Verification items for the finished model (mm, model axes). A direction names the side the tool comes from. Give positions to 0.01 mm unless a question says otherwise; leave off trailing zeros. Loops run counter-clockwise (first coordinate to the right, second up) from the corner with the lowest first, then second, coordinate; pieces in that order, holes last. Notation, with made-up numbers: M 89,70 L 104,70 A24 cw 104,107 Z; hole C 48.5,80 d5. An arc over 180 degrees is marked long. Use a Markdown table: item, result.
from build123d import *

# Parameters (mm, degrees)
F_2_6_MM_REMOVABLE_SHELF_WIRING_NOTC_2_R       = 1.65
F_2_6_MM_REMOVABLE_SHELF_WIRING_NOTC_2_R_2     = 1.15
F_2_6_MM_REMOVABLE_SHELF_WIRING_NOTCH_AN_DEPTH = 2.6
CONTROLLER_START                               = 2.6
CONTROLLER_BOARD_EDGE_RESTS_PROFILE_W          = 60
CONTROLLER_BOARD_EDGE_RESTS_PROFILE_H          = 1.6
CONTROLLER_BOARD_EDGE_RESTS_DEPTH              = 2


with BuildPart() as part:
    # 2.6 mm removable shelf - wiring notc 2 → 2.6 mm removable shelf - wiring notch an (new body)
    with BuildSketch(Plane.XY):
        Polygon((-41.9, -24.5), (41.9, -24.5), (41.9, 10.6), (20, 10.6), (20, 8.9), (-15, 8.9), (-15, 10.6), (-41.9, 10.6), (-41.9, -1), (-34, -1), (-34, -13), (-41.9, -13), align=None)
        with Locations((-38.8, -18.5)):
            Circle(F_2_6_MM_REMOVABLE_SHELF_WIRING_NOTC_2_R, mode=Mode.SUBTRACT)
        with Locations((38.8, -18.5)):
            Circle(F_2_6_MM_REMOVABLE_SHELF_WIRING_NOTC_2_R, mode=Mode.SUBTRACT)
        with Locations((-38.8, 2.5)):
            Circle(F_2_6_MM_REMOVABLE_SHELF_WIRING_NOTC_2_R, mode=Mode.SUBTRACT)
        with Locations((38.8, 2.5)):
            Circle(F_2_6_MM_REMOVABLE_SHELF_WIRING_NOTC_2_R, mode=Mode.SUBTRACT)
        with Locations((-23, -22.7)):
            Circle(F_2_6_MM_REMOVABLE_SHELF_WIRING_NOTC_2_R_2, mode=Mode.SUBTRACT)
        with Locations((25, -22.7)):
            Circle(F_2_6_MM_REMOVABLE_SHELF_WIRING_NOTC_2_R_2, mode=Mode.SUBTRACT)
        with Locations((-23, 8.7)):
            Circle(F_2_6_MM_REMOVABLE_SHELF_WIRING_NOTC_2_R_2, mode=Mode.SUBTRACT)
        with Locations((25, 8.7)):
            Circle(F_2_6_MM_REMOVABLE_SHELF_WIRING_NOTC_2_R_2, mode=Mode.SUBTRACT)
    extrude(amount=F_2_6_MM_REMOVABLE_SHELF_WIRING_NOTCH_AN_DEPTH)

    # Controller board edge rests profile → Controller board edge rests (add)
    with BuildSketch(Plane.XY.offset(CONTROLLER_START)):
        with Locations((0, -20.1)):
            Rectangle(CONTROLLER_BOARD_EDGE_RESTS_PROFILE_W, CONTROLLER_BOARD_EDGE_RESTS_PROFILE_H)
        with Locations((0, 6.1)):
            Rectangle(CONTROLLER_BOARD_EDGE_RESTS_PROFILE_W, CONTROLLER_BOARD_EDGE_RESTS_PROFILE_H)
    extrude(amount=CONTROLLER_BOARD_EDGE_RESTS_DEPTH)


solid = part.part
(1) Gauge pin test, flat ends, axial feed: P1, Ø5.5, axis at x = -38.8, y = -18.5, coming from the +Z side; P2, Ø1, axis at x = -0.5, z = 3.5, coming from the -Y side; P3, Ø1.5, axis at y = -11, z = 3, coming from the -X side; P4, Ø3, axis at x = 38.8, y = 2.5, coming from the +Z side. Record the tip position at first contact, or that the pin passes through.
Results below:
| item | result |
|---|---|
| P1 | z = 2.6 |
| P2 | y = -20.9 |
| P3 | x = -34 |
| P4 | through |
(2) Draft check along X on faces 4 (the cylindrical face through (-40.45, -18.43, 1.28)), 5 (the cylindrical face through (40.374, -18.004, 1.282)), 6 (the flat face through (-34, -7, 1)), 7 (the flat face through (-28, 10.6, 1)). Enter one of: +X half, -X half, draft (parallel to the pull), parting line (faces both ways), or undercut.
Results below:
| item | result |
|---|---|
| face 4 | undercut |
| face 5 | undercut |
| face 6 | -X half |
| face 7 | draft |
(3) Cross-section at B-B on z = 0.8. State how many separate pieces and enclosed holes the cut face has, then the cut area to 3 significant figures.
Results below:
| item | result |
|---|---|
| separate pieces | 1 |
| enclosed holes | 8 |
| area | 2,740 mm^2 |
(4) Cross-section at A-A on x = 38.8. Record the cut outline in (y, z), then the cut area to 3 significant figures.
Results below:
| item | result |
|---|---|
| outline | M -24.5,0 L -20.15,0 L -20.15,2.6 L -24.5,2.6 Z; M -16.85,0 L 0.85,0 L 0.85,2.6 L -16.85,2.6 Z; M 4.15,0 L 10.6,0 L 10.6,2.6 L 4.15,2.6 Z |
| area | 74.1 mm^2 |
(5) Cross-section at C-C on y = -22.7. Record the cut outline in (x, z), then the cut area to 3 significant figures.
Results below:
| item | result |
|---|---|
| outline | M -41.9,0 L -24.15,0 L -24.15,2.6 L -41.9,2.6 Z; M -21.85,0 L 23.85,0 L 23.85,2.6 L -21.85,2.6 Z; M 26.15,0 L 41.9,0 L 41.9,2.6 L 26.15,2.6 Z |
| area | 206 mm^2 |
(6) Set-up check for faces 1 (the flat face through (30, -20, 4)), 2 (the flat face through (-15, 10, 1)), 3 (the flat face through (0, -19.3, 4)): record each of +Z, -Z, +X, -X, +Y, -Y from which the full face is reachable in a straight line by a thin tool's end or side.
Results below:
| item | result |
|---|---|
| face 1 | +Z, +X, +Y, -Y |
| face 2 | +Z, -Z, +Y |
| face 3 | +Z, +X, -X |
(7) Cross-section at D-D on x = -38.8. Record the cut outline in (y, z), then the cut area to 3 significant figures.
Results below:
| item | result |
|---|---|
| outline | M -24.5,0 L -20.15,0 L -20.15,2.6 L -24.5,2.6 Z; M -16.85,0 L -13,0 L -13,2.6 L -16.85,2.6 Z; M -1,0 L 0.85,0 L 0.85,2.6 L -1,2.6 Z; M 4.15,0 L 10.6,0 L 10.6,2.6 L 4.15,2.6 Z |
| area | 42.9 mm^2 |
(8) Material ranges on line 1 (Y direction, x = -23, z = 0.5); line 2 (Y direction, x = -24.5, z = 3.25); line 3 (Z direction, x = 34, y = -3), recorded low to high.
Results below:
| item | result |
|---|---|
| line 1 | -24.5 to -23.85, -21.55 to 7.55, 9.85 to 10.6 |
| line 2 | -20.9 to -19.3, 5.3 to 6.9 |
| line 3 | 0 to 2.6 |
